CAD build for the part. Positions are in the model's coordinates, mm. Round coordinates to 2 decimals unless told otherwise and drop trailing zeros. Order: outer loops, then holes, each group sorted by start corner. A loop starts at its lowest first (then second) coordinate and runs counter-clockwise, first axis right, second up. Notation, with made-up numbers: M 64,14 L 117,14 A8 cw 117,27 Z; hole C 34,24.5 d10. An arc over 180 degrees is marked long. Answer as a JSON object with one key per item and string values. Group by question number.
```python
from build123d import *

# Parameters (mm, degrees)
SKETCH1_R           = 47.5
SKETCH1_R_2         = 2
BOSS_EXTRUDE1_DEPTH = 5


with BuildPart() as part:
    # Sketch1 → Boss-Extrude1 (new body)
    with BuildSketch(Plane(origin=(0, 0, 0), x_dir=(1, 0, 0), z_dir=(0, 1, 0))):
        Circle(SKETCH1_R)
        with Locations((0, 42.5)):
            Circle(SKETCH1_R_2, mode=Mode.SUBTRACT)
        with Locations((40.419901943, 13.133222261)):
            Circle(SKETCH1_R_2, mode=Mode.SUBTRACT)
        with Locations((24.980873222, -34.383222261)):
            Circle(SKETCH1_R_2, mode=Mode.SUBTRACT)
        with Locations((-24.980873222, -34.383222261)):
            Circle(SKETCH1_R_2, mode=Mode.SUBTRACT)
        with Locations((-40.419901943, 13.133222261)):
            Circle(SKETCH1_R_2, mode=Mode.SUBTRACT)
    extrude(amount=BOSS_EXTRUDE1_DEPTH)


solid = part.part
```
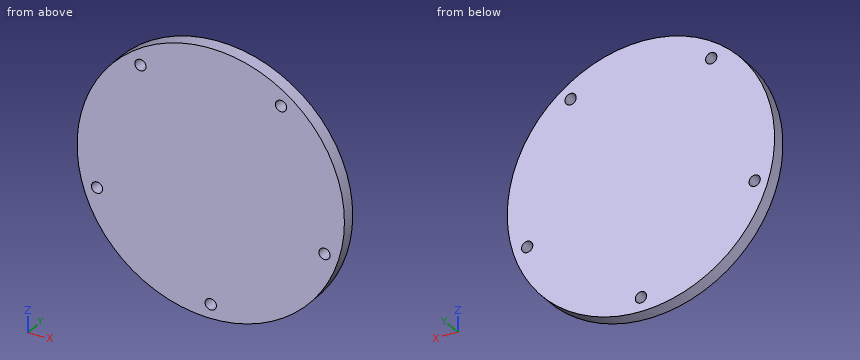
Item 1: Cut at B-B, the plane z = -42.5. Give the cut face in (x, y), and give its area (3 significant figures).
Item 2: Cut at A-A, the plane x = 0. Give the cut face in (y, z).
Item 3: Drill centre lines: line 1 (Z direction, x = 0, y = 2.35); line 2 (X direction, y = 2.65, z = 0.5); line 3 (X direction, y = 1.65, z = -42.5). Where is each one in solid material? Low to high. Write a range as [from, to].
Item 4: Cut at C-C, the plane y = 3.75. Give the cut face in (x, z), and give its area (3 significant figures).
Item 5: Flat gauge pins, fed straight in: pin 1 Ø6 at (x, z) = (-5.5, -14) entering from -Y; pin 2 Ø2 at (y, z) = (2.5, -14) entering from -X; pin 3 Ø1.5 at (y, z) = (1.5, -29.5) entering from +X. Where does each tip first touch, or does it go through?
Item 6: Cut at D-D, the plane x = 10. Give the cut face in (y, z).
Response values:
{
 "1": {"outline": "M -21.21,0 L -2,0 L -2,5 L -21.21,5 Z; M 2,0 L 21.21,0 L 21.21,5 L 2,5 Z", "area": "192 mm^2"},
 "2": {"outline": "M 0,-47.5 L 5,-47.5 L 5,-44.5 L 0,-44.5 Z; M 0,-40.5 L 5,-40.5 L 5,47.5 L 0,47.5 Z"},
 "3": {"line 1": "[-47.5, -44.5], [-40.5, 47.5]", "line 2": "[-47.5, 47.5]", "line 3": "[-21.21, -2], [2, 21.21]"},
 "4": {"outline": "C 0,0 d95; hole C -40.42,-13.13 d4; hole C -24.98,34.38 d4; hole C 0,-42.5 d4; hole C 24.98,34.38 d4; hole C 40.42,-13.13 d4", "area": "7,030 mm^2"},
 "5": {"pin 1": "y = 0", "pin 2": "x = -45.69", "pin 3": "x = 37.81"},
 "6": {"outline": "M 0,-46.44 L 5,-46.44 L 5,46.44 L 0,46.44 Z"}
}
